from build123d import *

# Parameters (mm, degrees)
F0_W     = 400
F0_H     = 352
F1_DEPTH = 19
F3_DEPTH = 19.001
F4_R     = 17.0766139483
F5_DEPTH = 19.0010001


with BuildPart() as f1:
    # F0 (on Top) → F1 (new body)
    with BuildSketch(Plane.XY):
        Rectangle(F0_W, F0_H)
    extrude(amount=F1_DEPTH)

    # F2 (on face) → F3 (cut, through all)
    with BuildSketch(Plane.XY.offset(19)):
        with BuildLine():
            add(Edge.make_bspline(
                [(-200, -78.359618783), (-195.7803636721, -92.9464094347), (-188.2077942368, -119.1238987881), (-172.8338241624, -143.2121066887), (-156.2569923786, -165.3855569544), (-115.975253997, -175.3258984721), (-115.6307756901, -176)],
                knots=[0, 0, 0, 0, 0.2648009651, 0.4752124447, 0.7001594462, 0.9450581233, 0.9450581233, 0.9450581233, 0.9450581233], degree=3))
            Line((-200, -78.359618783), (-200, -176))
            Line((-200, -176), (-117.4777597189, -176))
            Line((-117.4777597189, -176), (-115.6307756901, -176))
        make_face()
        with BuildLine():
            Line((200, 176), (111.9655743241, 176))
            add(Edge.make_bspline(
                [(111.9655743241, 176), (123.0835042522, 170.3676733426), (145.2416377316, 159.1423960938), (172.7110494727, 144.455694766), (198.7014382707, 79.4978346928), (200, 73.2613801956)],
                knots=[0, 0, 0, 0, 0.2786310963, 0.5553142594, 0.9453657408, 0.9453657408, 0.9453657408, 0.9453657408], degree=3))
            Line((200, 73.2613801956), (200, 176))
        make_face()
    extrude(amount=-F3_DEPTH, mode=Mode.SUBTRACT)

    # F4 (on face) → F5 (cut, through all)
    with BuildSketch(Plane.XY.offset(19)):
        with Locations((-138.4022831917, -123.3757436275)):
            Circle(F4_R)
    extrude(amount=-F5_DEPTH, mode=Mode.SUBTRACT)


solid = f1.part
Input: part model. Units: mm. Frame: model coordinates. Coordinates: 2 decimals unless noted, no trailing zeros.
Q1. Draft query along X for faces 1 (the face through (-3, 2, 19)), 2 (the face through (200, -53, 9)), 3 (the face through (-142.104, -140.046, 9.633)), 4 (the face through (-200, 47, 9)). Return one class per face: +X half, -X half, draft (parallel to the pull), parting line (faces both ways), or undercut.
Q2. Material intervals for line 1 (X direction, y = -122, z = 6.25); line 2 (X direction, y = -131.5, z = 12.5); line 3 (Y direction, x = 149.5, z = 10.75), sorted ascending.
Q3. Contact query for a flat-ended pin moving along its axis: pin 1 (3 mm diameter, centred on y = 132, z = 12.5, fed in from +X). Output: stop coordinate, or through.
Working result:
1. face 1: draft
1. face 2: +X half
1. face 3: undercut
1. face 4: -X half
2. line 1: x = -185.11 to -155.42, -121.38 to 200
2. line 2: x = -180.04 to -153.42, -123.38 to 200
2. line 3: y = -176 to 156.71
3. pin 1: stops at x = 174.5
